Check sheet for the modelled part. Datum: model origin and axes. Units: mm. Face numbers are marked on the shaded views. A direction names the side the tool comes from. Round coordinates to 2 decimals unless told otherwise and drop trailing zeros. Order: outer loops, then holes, each group sorted by start corner. A loop starts at its lowest first (then second) coordinate and runs counter-clockwise, first axis right, second up.
Q1. Cross-section at A-A on y = 2. Record the cut outline in (x, z), then the cut area to 3 significant figures.
Q2. Cross-section at C-C on y = 13.5. Record the cut outline in (x, z), then the cut area to 3 significant figures.
Q3. Mould release check, pull along Y, two halves, no side actions. Record for the marked faces 1, 2 and 3: +Y half, -Y half, draft (parallel to the pull), parting line (faces both ways), or undercut.
Q4. Cross-section at B-B on x = 5. Record the cut outline in (y, z), then the cut area to 3 significant figures.
Q5. Set-up check for the marked faces 4, 5 and 6: record each of +Z, -Z, +X, -X, +Y, -Y from which the full face is reachable in a straight line by a thin tool's end or side.
Q6. Scan lines: probe 1 along X at (y, z) = (10, 5.5); probe 2 along Y at (x, z) = (35, 7.5); probe 3 along X at (y, z) = (-11.5, 4.75). Record each from-to range of solid material in increasing order.
Q7. Depth check by flat-ended pin: P1, Ø4, axis at y = -10.5, z = 2, coming from the -X side. Enter the tip coordinate at first touch or a pass-through.
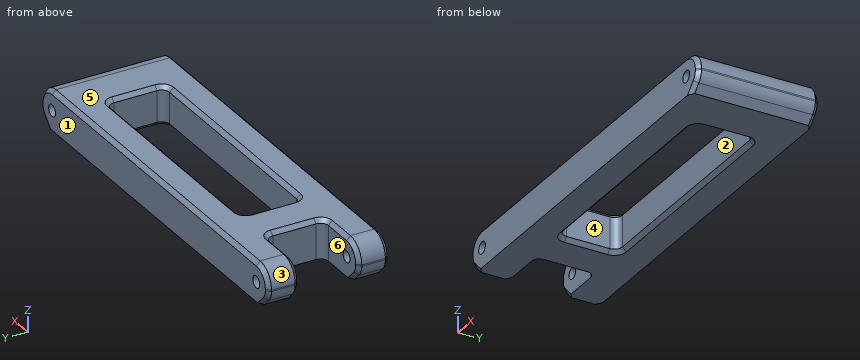
from build123d import *

# Parameters (mm, degrees)
F0_W     = 60
F0_H     = 15
F1_DEPTH = 10
F2_R     = 5
F3_SIZE  = 3
F4_R     = 4
F5_R     = 2
F6_R     = 1.5
F7_DEPTH = 31.001
F8_SIZE  = 1


with BuildPart() as f1:
    # F0 (on Top) → F1 (new body)
    with BuildSketch(Plane.XY):
        Polygon((-23.9456994958, 15.5), (-23.9456994958, 7.5), (-8.9456994958, 7.5), (-8.9456994958, -7.5), (-23.9456994958, -7.5), (-23.9456994958, -15.5), (76.0543005042, -15.5), (76.0543005042, 15.5), align=None)
        with Locations((31.0543005042, 0)):
            Rectangle(F0_W, F0_H, mode=Mode.SUBTRACT)
    extrude(amount=F1_DEPTH)

    # F2
    f2_edges = [f1.edges().sort_by_distance(p)[0] for p in [
        (-23.945699, 11.5, 10),
        (-23.945699, -11.5, 10),
        (76.054301, 0, 10),
    ]]
    fillet(f2_edges, radius=F2_R)

    # F3
    f3_edges = [f1.edges().sort_by_distance(p)[0] for p in [
        (-23.945699, 11.5, 0),
        (-23.945699, -11.5, 0),
        (76.054301, 0, 0),
    ]]
    chamfer(f3_edges, length=F3_SIZE)

    # F4
    f4_edges = [f1.edges().sort_by_distance(p)[0] for p in [
        (76.054301, 0, 3),
        (-23.945699, -11.5, 3),
        (-23.945699, 11.5, 3),
    ]]
    fillet(f4_edges, radius=F4_R)

    # F5
    f5_edges = [f1.edges().sort_by_distance(p)[0] for p in [
        (-8.945699, 7.5, 5),
        (-8.945699, -7.5, 5),
        (1.054301, 7.5, 5),
        (1.054301, -7.5, 5),
        (61.054301, 7.5, 5),
        (61.054301, -7.5, 5),
    ]]
    fillet(f5_edges, radius=F5_R)

    # F6 (on face) → F7 (cut, through all)
    with BuildSketch(Plane.XZ.offset(15.5)):
        with Locations((-18.9456994958, 5)):
            Circle(F6_R)
        with Locations((71.0543005042, 5)):
            Circle(F6_R)
    extrude(amount=-F7_DEPTH, mode=Mode.SUBTRACT)

    # F8
    f8_edges = [f1.edges().sort_by_distance(p)[0] for p in [
        (-14.945699, 7.5, 10),
        (26.054301, 15.5, 10),
        (31.054301, 7.5, 10),
        (31.054301, 7.5, 0),
        (26.054301, -15.5, 10),
    ]]
    chamfer(f8_edges, length=F8_SIZE)


solid = f1.part
Results found:
1. outline: (-8.95, 0) - (0.05, 0) - (1.05, 1) - (1.05, 9) - (0.05, 10) - (-7.95, 10) - (-8.95, 9) - close; (61.05, 1) - (62.05, 0) - (73.05, 0) - (74.88, 1.83) arc R4 ccw to (76.05, 4.66) - (76.05, 5) arc R5 ccw to (71.05, 10) - (62.05, 10) - (61.05, 9) - close; hole circle Ø3 at (71.05, 5)
1. area: 230 mm2
2. outline: (-23.95, 4.66) arc R4 ccw to (-22.77, 1.83) - (-20.95, 0) - (73.05, 0) - (74.88, 1.83) arc R4 ccw to (76.05, 4.66) - (76.05, 5) arc R5 ccw to (71.05, 10) - (-18.95, 10) arc R5 ccw to (-23.95, 5) - close; hole circle Ø3 at (-18.95, 5); hole circle Ø3 at (71.05, 5)
2. area: 965 mm2
3. face 1: +Y half
3. face 2: undercut
3. face 3: draft
4. outline: (-15.5, 0) - (-8.5, 0) - (-7.5, 1) - (-7.5, 9) - (-8.5, 10) - (-14.5, 10) - (-15.5, 9) - close; (7.5, 1) - (8.5, 0) - (15.5, 0) - (15.5, 9) - (14.5, 10) - (8.5, 10) - (7.5, 9) - close
4. area: 157 mm2
5. face 4: +Z, -Z
5. face 5: +Z, +X, -X, +Y, -Y
5. face 6: +Z, -Z, -X
6. probe 1: x = -23.92 to -20.36, -17.53 to 69.64, 72.47 to 76.03
6. probe 2: y = -15.5 to -7.5, 7.5 to 15.5
6. probe 3: x = -23.95 to -20.42, -17.47 to 69.58, 72.53 to 76.05
7. P1: stops at x = -23.89
